Answer from the drawing. Dimensions are ordinates in mm from the lowest x, y and z of the part. A direction names the side the tool comes from. Coordinates: 2 decimals unless noted, no trailing zeros. Loops run counter-clockwise (first coordinate to the right, second up) from the corner with the lowest first, then second, coordinate; pieces in that order, holes last. Notation, with made-up numbers: (-8.5, -35) -> (27.5, -35) arc R7 ccw to (27.5, -25) -> close; hole circle Ø6 at (-23.5, 55). An arc over 180 degrees is marked (long way). Use a Markdown table: item, result.
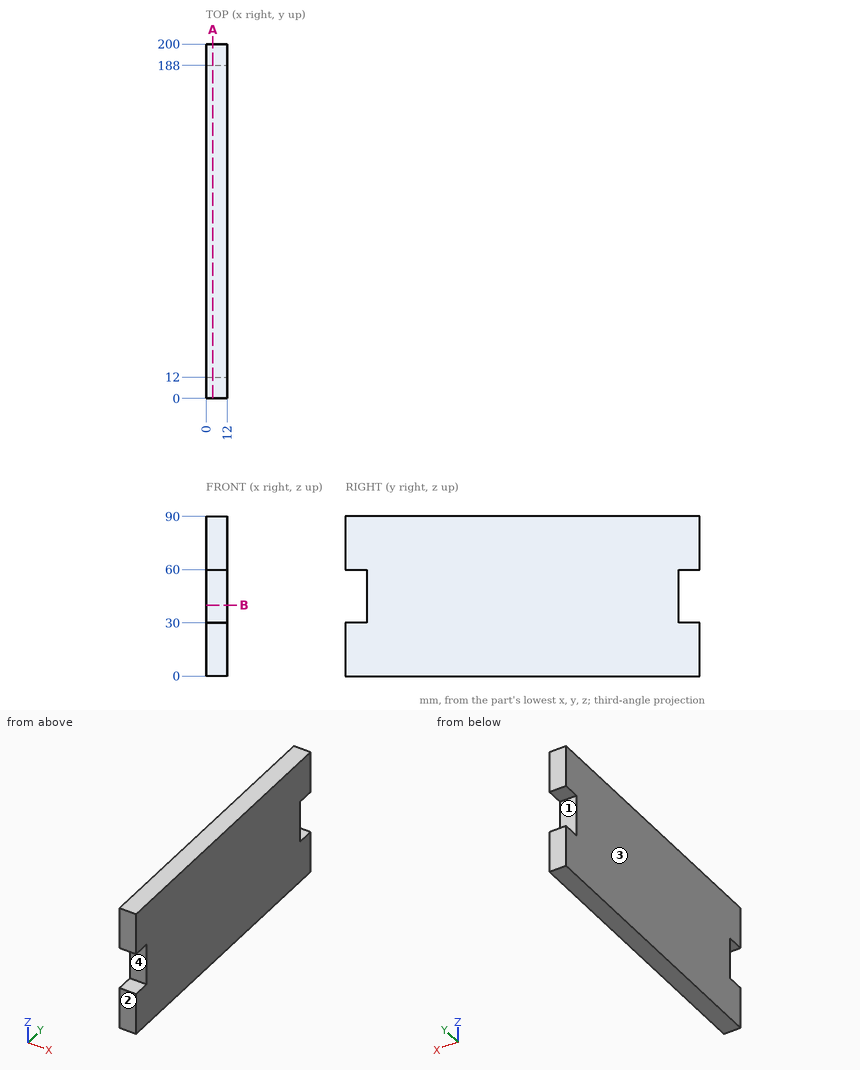
Q1. Given pin 1 Ø4 at (x, z) = (7.5, 45.5) entering from +Y; pin 2 Ø6 at (x, z) = (5.5, 47) entering from -Y, each flat-ended and moving along its own axis, determine where each tip first touches the part or whether it passes through.
Solved:
| item | result |
|---|---|
| pin 1 | y = 188 |
| pin 2 | y = 12 |
Q2. Section A-A on x = 3.75 is taken. Determine the outline of the cut face in (y, z).
Solved:
| item | result |
|---|---|
| outline | (0, 0) -> (200, 0) -> (200, 30) -> (188, 30) -> (188, 60) -> (200, 60) -> (200, 90) -> (0, 90) -> (0, 60) -> (12, 60) -> (12, 30) -> (0, 30) -> close |
Q3. Consider line 1 (Y direction, x = 1.75, z = 41). Determine where the line is inside the solid, lowest interval first. Write a range as [from, to].
Solved:
| item | result |
|---|---|
| line 1 | [12, 188] |
Q4. Section B-B on z = 40 is taken. Determine the outline of the cut face in (x, y), and give its area (3 significant figures).
Solved:
| item | result |
|---|---|
| outline | (0, 12) -> (12, 12) -> (12, 188) -> (0, 188) -> close |
| area | 2,110 mm² |
Q5. For the marked faces 3 and 4, determine the directions among +Z, -Z, +X, -X, +Y, -Y from which every point of the face is accessible in a straight line to the end or side of a thin tool.
Solved:
| item | result |
|---|---|
| face 3 | +Z, -Z, -X, +Y, -Y |
| face 4 | +X, -X, -Y |
Q6. Determine the mould class of the marked faces 1 and 2 for opening direction Z: pulls with the +Z half, pulls with the -Z half, needs draft (parallel to the pull), parting line crosses it, or undercut.
Solved:
| item | result |
|---|---|
| face 1 | undercut |
| face 2 | needs draft |
